from build123d import *

# Parameters (mm, degrees)
F0_W     = 84
F0_H     = 61
F1_DEPTH = 84
F2_R     = 8
F3_T     = -3
F4_R     = 6.35
F5_DEPTH = 2
F6_R     = 6.35
F7_DEPTH = 2
F8_W     = 40
F8_H     = 40
F9_DEPTH = 50


with BuildPart() as f1:
    # F0 (on Top) → F1 (new body)
    with BuildSketch(Plane.XY):
        Rectangle(F0_W, F0_H)
    extrude(amount=F1_DEPTH)

    # F2
    f2_edges = [f1.edges().sort_by_distance(p)[0] for p in [
        (-42, 0, 84),
        (-42, 30.5, 42),
        (0, 30.5, 84),
        (0, 30.5, 0),
        (-42, 0, 0),
        (42, 0, 84),
        (42, 30.5, 42),
        (42, 0, 0),
    ]]
    fillet(f2_edges, radius=F2_R)

    # F3
    f3_openings = [f1.faces().sort_by_distance(p)[0] for p in [
        (0, -30.5, 42),
    ]]
    offset(amount=F3_T, openings=f3_openings)

    # F4 (on face) → F5 (join)
    with BuildSketch(Plane.XY.offset(3)):
        with Locations((0, -1.681145)):
            Circle(F4_R)
    extrude(amount=F5_DEPTH)

    # F6 (on face) → F7 (join)
    with BuildSketch(Plane(origin=(39, 0, 0), x_dir=(0, -1, 0), z_dir=(-1, 0, 0))):
        with Locations((0, 42)):
            Circle(F6_R)
    extrude(amount=F7_DEPTH)

    # F8 (on face) → F9 (join)
    with BuildSketch(Plane.XZ.offset(-27.5)):
        with Locations((-9, 51)):
            Rectangle(F8_W, F8_H)
    extrude(amount=F9_DEPTH)


solid = f1.part
Source: CAD feature listing. Evaluate the final solid. Frame: model axes, mm. A direction names the side the tool comes from. Give positions to 0.01 mm unless a question says otherwise; leave off trailing zeros. Write each loop counter-clockwise with the first axis right and the second up, starting at its lowest first coordinate (ties: lowest second). Pieces come first, ordered by that corner, then holes. Notation, with made-up numbers: (-19.75, -30.75) -> (-7.75, -30.75) arc R31 cw to (-7.75, 1.25) -> close; hole circle Ø2 at (36.25, 68). An arc over 180 degrees is marked (long way). Write item = value, one per line.
Q1. Cut plane D-D on y = -3. Return loops of the section in (x, z).
Here are the results:
outline = (-42, 8) arc R8 ccw to (-34, 0) -> (34, 0) arc R8 ccw to (42, 8) -> (42, 76) arc R8 ccw to (34, 84) -> (-34, 84) arc R8 ccw to (-42, 76) -> close; (-29, 31) -> (11, 31) -> (11, 71) -> (-29, 71) -> close; hole (-39, 8) arc R5 ccw to (-34, 3) -> (-6.21, 3) -> (-6.21, 5) -> (6.21, 5) -> (6.21, 3) -> (34, 3) arc R5 ccw to (39, 8) -> (39, 36.4) -> (37, 36.4) -> (37, 47.6) -> (39, 47.6) -> (39, 76) arc R5 ccw to (34, 81) -> (-34, 81) arc R5 ccw to (-39, 76) -> close
Q2. First-contact query: pin 1 (3 mm diameter, centred on x = -1.5, z = 24, fed in from -Y); pin 2 (20 mm diameter, centred on x = -17, z = 44, fed in from -Y). Flat tips, straight axial feed; report the tip coordinate or a pass-through.
Here are the results:
pin_1 = 27.5
pin_2 = -22.5
Q3. Line query: line 1 (X direction, y = 5, z = 33); line 2 (Z direction, x = -23, y = -4); line 3 (X direction, y = 14, z = 76). Output: solid intervals per line, ascending. Write a range as from..to.
Here are the results:
line_1 = -42..-39, -29..11, 39..42
line_2 = 0..3, 31..71, 81..84
line_3 = -42..-39, 39..42
Q4. Cut plane C-C on x = 0. Return loops of the section in (y, z), then the cut area to 3 significant figures.
Here are the results:
outline = (-30.5, 0) -> (22.5, 0) arc R8 ccw to (30.5, 8) -> (30.5, 76) arc R8 ccw to (22.5, 84) -> (-30.5, 84) -> (-30.5, 81) -> (22.5, 81) arc R5 cw to (27.5, 76) -> (27.5, 71) -> (-22.5, 71) -> (-22.5, 31) -> (27.5, 31) -> (27.5, 8) arc R5 cw to (22.5, 3) -> (4.67, 3) -> (4.67, 5) -> (-8.03, 5) -> (-8.03, 3) -> (-30.5, 3) -> close
area = 2,610 mm²
Q5. Cut plane B-B on z = 42. Return loops of the section in (x, y).
Here are the results:
outline = (-42, -30.5) -> (-39, -30.5) -> (-39, 22.5) arc R5 cw to (-34, 27.5) -> (-29, 27.5) -> (-29, -22.5) -> (11, -22.5) -> (11, 27.5) -> (34, 27.5) arc R5 cw to (39, 22.5) -> (39, 6.35) -> (37, 6.35) -> (37, -6.35) -> (39, -6.35) -> (39, -30.5) -> (42, -30.5) -> (42, 22.5) arc R8 ccw to (34, 30.5) -> (-34, 30.5) arc R8 ccw to (-42, 22.5) -> close
Q6. Reachability of faces 4 (the face through (-39.719, -3.629, 2.406)), 5 (the face through (-37.57, 26, 42.48)), 6 (the face through (38.01, 1.38, 35.8)) from +Z, -Z, +X, -X, +Y, -Y: full face, straight path, thin tool, end or side. Return the list, or none.
Here are the results:
face_4 = -Z, -X, +Y, -Y
face_5 = -Y
face_6 = none
Q7. Mould query, pull axis Z, two halves, no side actions, for faces 1 (the face through (-38, -4, 5)), 2 (the face through (0, -30.5, 1)), 3 (the face through (0, -4, 0)). Classes: +Z half, -Z half, draft (parallel to the pull), parting line (faces both ways), or undercut.
Here are the results:
face_1 = undercut
face_2 = draft
face_3 = -Z half
Q8. Cut plane A-A on y = -14.5. Return loops of the section in (x, z).
Here are the results:
outline = (-42, 8) arc R8 ccw to (-34, 0) -> (34, 0) arc R8 ccw to (42, 8) -> (42, 76) arc R8 ccw to (34, 84) -> (-34, 84) arc R8 ccw to (-42, 76) -> close; (-29, 31) -> (11, 31) -> (11, 71) -> (-29, 71) -> close; hole (-39, 8) arc R5 ccw to (-34, 3) -> (34, 3) arc R5 ccw to (39, 8) -> (39, 76) arc R5 ccw to (34, 81) -> (-34, 81) arc R5 ccw to (-39, 76) -> close
